from build123d import *

# Parameters (mm, degrees)
F0_W     = 20
F0_H     = 30
F1_DEPTH = 4
F2_W     = 3.8
F2_H     = 30
F3_DEPTH = 20
F5_DEPTH = 25
F6_R     = 3
F7_DEPTH = 25


with BuildPart() as f1:
    # F0 (on Front) → F1 (new body)
    with BuildSketch(Plane.XZ):
        Rectangle(F0_W, F0_H)
    extrude(amount=-F1_DEPTH)

    # F2 (on face) → F3 (join)
    with BuildSketch(Plane(origin=(0, 4, 0), x_dir=(-1, 0, 0), z_dir=(0, 1, 0))):
        with Locations((-8.1, 0)):
            Rectangle(F2_W, F2_H)
        with Locations((8.1, 0)):
            Rectangle(F2_W, F2_H)
        Rectangle(F2_W, F2_H)
    extrude(amount=F3_DEPTH)

    # F4 (on face) → F5 (cut)
    with BuildSketch(Plane.YZ.offset(10)):
        with BuildLine():
            ThreePointArc((9, 15), (19.606602, 10.606602), (24, 0))
            Line((24, 0), (24, 15))
            Line((24, 15), (9, 15))
        make_face()
        with BuildLine():
            Line((24, -15), (24, 0))
            ThreePointArc((24, 0), (19.606602, -10.606602), (9, -15))
            Line((9, -15), (24, -15))
        make_face()
    extrude(amount=-F5_DEPTH, mode=Mode.SUBTRACT)

    # F6 (on face) → F7 (cut)
    with BuildSketch(Plane.YZ.offset(10)):
        with Locations((16, 0)):
            Circle(F6_R)
    extrude(amount=-F7_DEPTH, mode=Mode.SUBTRACT)


solid = f1.part
Work out the finished part from the listing and answer in its coordinate system (mm). A direction names the side the tool comes from. Round coordinates to 2 decimals unless told otherwise and drop trailing zeros. Loops run counter-clockwise (first coordinate to the right, second up) from the corner with the lowest first, then second, coordinate; pieces in that order, holes last. Notation, with made-up numbers: (74, -31) - (119, -31) arc R25 ccw to (119, -2) - close; hole circle Ø11 at (34, -9.5). An arc over 180 degrees is marked (long way). Use one line per item in the form item = value. Start each with the question number.
(1) Find section A-A on y = 21. Determine the outline of the cut face in (x, z), and give its area (3 significant figures).
(2) Which of the six approach directions +Z, -Z, +X, -X, +Y, -Y give full straight-line access (tool end or side, diameter ignored) to faces 5 (the face through (0, 0, 0)), 6 (the face through (6.2, 12, 0))?
(3) Consider line 1 (X direction, y = 10.25, z = 11.5); line 2 (Y direction, x = -6, z = -4.5); line 3 (Z direction, x = 8, y = 16). Determine where each line is inside the solid, lowest interval first.
(4) Determine the mould class of faces 1 (the face through (8, 13, 0)), 2 (the face through (-8, 13, 0)), 3 (the face through (-1.9, 12, 0)), 4 (the face through (4, 4, 0)) for opening direction Y: +Y half, -Y half, draft (parallel to the pull), parting line (faces both ways), or undercut.
(5) Find section B-B on z = -12. Determine the outline of the cut face in (x, y), and give its area (3 significant figures).
(6) Flat-ended cylindrical pins translate along their axes: P1, Ø1.3, axis at x = -5, z = 7, coming from the +Y side; P2, Ø1, axis at x = -4, y = 21, coming from the -Z side; P3, Ø2, axis at x = 5.5, y = 18.5, coming from the -Z side; P4, Ø6, axis at x = -3, z = 6, coming from the +Y side. Find the tip coordinate at first contact, or state that the pin passes through.
(7) Find section C-C on x = 1.25. Determine the outline of the cut face in (y, z).
(8) Find section D-D on z = -2. Determine the outline of the cut face in (x, y), and give its area (3 significant figures).
Answer list:
q1.outline = (-10, -9) - (-6.2, -9) - (-6.2, 9) - (-10, 9) - close; (-1.9, -9) - (1.9, -9) - (1.9, 9) - (-1.9, 9) - close; (6.2, -9) - (10, -9) - (10, 9) - (6.2, 9) - close
q1.area = 205 mm^2
q2.face_5 = +Z, -Z, +X, -X, -Y
q2.face_6 = +Z, -Z, +Y
q3.line_1 = -10 to -6.2, -1.9 to 1.9, 6.2 to 10
q3.line_2 = 0 to 4
q3.line_3 = -13.27 to -3, 3 to 13.27
q4.face_1 = undercut
q4.face_2 = undercut
q4.face_3 = draft
q4.face_4 = +Y half
q5.outline = (-10, 0) - (10, 0) - (10, 18) - (6.2, 18) - (6.2, 4) - (1.9, 4) - (1.9, 18) - (-1.9, 18) - (-1.9, 4) - (-6.2, 4) - (-6.2, 18) - (-10, 18) - close
q5.area = 240 mm^2
q6.P1 = 4
q6.P2 = through
q6.P3 = -12.16
q6.P4 = 23.65
q7.outline = (0, -15) - (9, -15) arc R15 ccw to (24, 0) arc R15 ccw to (9, 15) - (0, 15) - close; hole circle Ø6 at (16, 0)
q8.outline = (-10, 0) - (10, 0) - (10, 13.76) - (6.2, 13.76) - (6.2, 4) - (1.9, 4) - (1.9, 13.76) - (-1.9, 13.76) - (-1.9, 4) - (-6.2, 4) - (-6.2, 13.76) - (-10, 13.76) - close; (-10, 18.24) - (-6.2, 18.24) - (-6.2, 23.87) - (-10, 23.87) - close; (-1.9, 18.24) - (1.9, 18.24) - (1.9, 23.87) - (-1.9, 23.87) - close; (6.2, 18.24) - (10, 18.24) - (10, 23.87) - (6.2, 23.87) - close
q8.area = 255 mm^2
